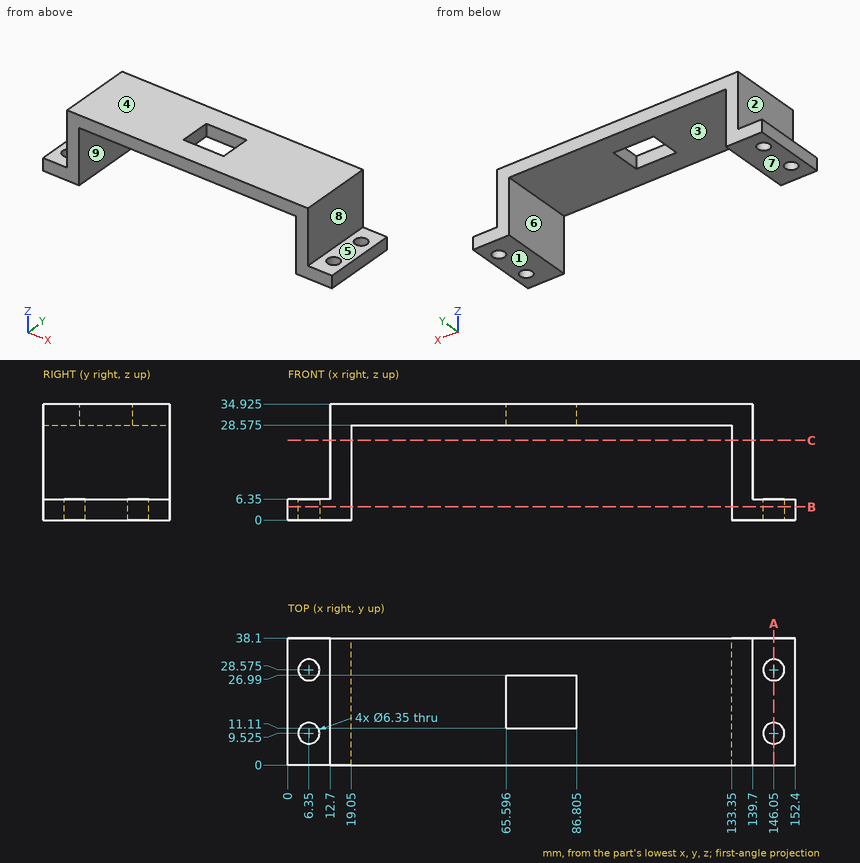
The figure shows three views and two pictorial views of one solid part (mm, origin at its lowest corner). Answer the questions. A direction names the side the tool comes from. Give positions to 0.01 mm unless a question says otherwise; leave off trailing zeros. Write each loop counter-clockwise with the first axis right and the second up, starting at its lowest first coordinate (ties: lowest second). Pieces come first, ordered by that corner, then holes. Notation, with made-up numbers: (50.25, 57) - (95.25, 57) arc R4 ccw to (95.25, 63) - close; hole circle Ø6 at (79, 58). An arc over 180 degrees is marked (long way). Use CSV: the item, a comma, the result in double quotes. Start each with the question number.
Item 1: Flat-ended cylindrical pins translate along their axes: P1, Ø10, axis at x = 146.05, y = 28.575, coming from the +Z side; P2, Ø6, axis at x = 110.5, y = 15.5, coming from the -Z side (1 decimal); P3, Ø7, axis at y = 17.5, z = 32.5, coming from the -X side. Find the tip coordinate at first contact, or state that the pin passes through.
Item 2: For the marked faces 1, 2, 3, 4 and 5, determine the directions among +Z, -Z, +X, -X, +Y, -Y from which every point of the face is accessible in a straight line to the end or side of a thin tool.
Item 3: Consider line 1 (Y direction, x = 146.05, z = 2); line 2 (X direction, y = 21, z = 11); line 3 (X direction, y = 11, z = 6). Determine where each line is inside the solid, lowest interval first.
Item 4: The mould has two halves that part along X. Classify the marked faces 6, 7, 8 and 9: pulls with the +X half, pulls with the -X half, needs draft (parallel to the pull), parting line crosses it, or undercut.
Item 5: The part is cut by section A-A, the plane x = 146.05. Give the vertices of the cut face in (y, z), and give its area (3 significant figures).
Item 6: The part is cut by section C-C, the plane z = 24. Give the vertices of the cut face in (x, y), and give its area (3 significant figures).
Item 7: The part is cut by section B-B, the plane z = 4. Count the separate pieces of the cut face and the enclosed holes in it, and give its area (4 significant figures).
Taken from the geometry:
1,P1,"z = 6.35"
1,P2,"z = 28.6"
1,P3,"x = 12.7"
2,face 1,"-Z, +X, -X, +Y, -Y"
2,face 2,"+Z, -X, +Y, -Y"
2,face 3,"-Z, +Y, -Y"
2,face 4,"+Z, +X, -X, +Y, -Y"
2,face 5,"+Z, +X, +Y, -Y"
3,line 1,"0 to 6.35, 12.7 to 25.4, 31.75 to 38.1"
3,line 2,"12.7 to 19.05, 133.35 to 139.7"
3,line 3,"0 to 3.54, 9.16 to 19.05, 133.35 to 143.24, 148.86 to 152.4"
4,face 6,"undercut"
4,face 7,"needs draft"
4,face 8,"pulls with the +X half"
4,face 9,"undercut"
5,outline,"(0, 0) - (6.35, 0) - (6.35, 6.35) - (0, 6.35) - close; (12.7, 0) - (25.4, 0) - (25.4, 6.35) - (12.7, 6.35) - close; (31.75, 0) - (38.1, 0) - (38.1, 6.35) - (31.75, 6.35) - close"
5,area,"161 mm2"
6,outline,"(12.7, 0) - (19.05, 0) - (19.05, 38.1) - (12.7, 38.1) - close; (133.35, 0) - (139.7, 0) - (139.7, 38.1) - (133.35, 38.1) - close"
6,area,"484 mm2"
7,separate pieces,"2"
7,enclosed holes,"4"
7,area,"1,325 mm2"
